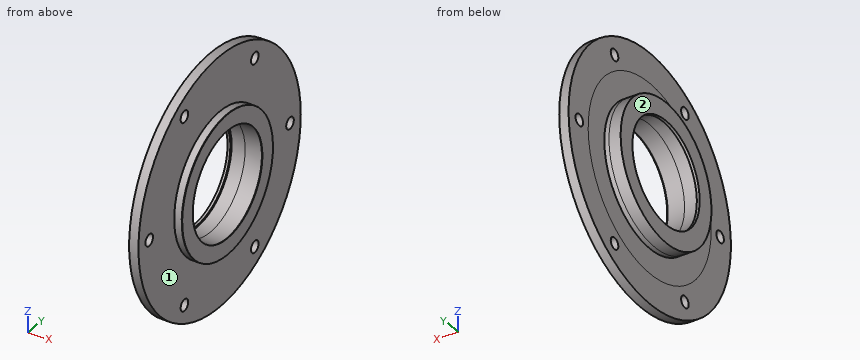
Autodesk Inventor part; units mm, degrees
ref_plane "Work Plane1" through (-10, 0, 0) normal (-1, 0, 0) x (0, 0, 1)
ref_plane "YZ Plane" through (0, 0, 0) normal (1, 0, 0) x (0, 1, 0)
ref_plane "XZ Plane" through (0, 0, 0) normal (0, 1, 0) x (-1, 0, 0)
sketch "Sketch1" plane through (0, 0, 0) normal (1, 0, 0) x (0, 1, 0)
  circle A0 centre (0, 0) radius 268
  circle A1 centre (0, 0) radius 203.25
  circle A2 centre (0, 0) radius 232.5
  circle A3 centre (232.5, 0) radius 12.5
  circle A4 centre (116.25, 201.3509) radius 12.5
  circle A5 centre (-116.25, 201.3509) radius 12.5
  circle A6 centre (-232.5, 0) radius 12.5
  circle A7 centre (-116.25, -201.3509) radius 12.5
  circle A8 centre (116.25, -201.3509) radius 12.5
  dimension "d2" = 465
  dimension "d0" = 536
  dimension "d1" = 406.5
  dimension "d3" = 25
  dimension "d101" = 360
extrude "Extrusion1" add sketch "Sketch1" along normal blind 20 contours A0 | A3 A2 A8 A7 A6 A5 A4
sketch "Sketch2" plane through (0, 0, 0) normal (1, 0, 0) x (0, 1, 0)
  circle A0 centre (0, 0) radius 115
  circle A1 centre (0, 0) radius 150
  dimension "d10" = 230
  dimension "d11" = 300
extrude "Extrusion2" add sketch "Sketch2" against normal mid plane 70
ref_plane "Work Plane1" through (-10, 0, 0) normal (-1, 0, 0) x (0, 0, 1)
sketch "Sketch3" plane through (-10, 0, 0) normal (-1, 0, 0) x (0, 0, 1)
  circle A0 centre (0, 0) radius 203.25
  circle A1 centre (0, 0) radius 150
  dimension "d15" = 406.5
  dimension "d16" = 300
extrude "Extrusion3" add sketch "Sketch3" against normal blind 30
sketch "Sketch4" plane through (-35, 0, 0) normal (-1, 0, 0) x (0, 0, 1)
  circle A0 centre (0, 0) radius 113.4667
  circle A1 centre (0, 0) radius 111
  circle A2 centre (0, 0) radius 115
  dimension "d43" = 222
  dimension "d44" = 230
extrude "Extrusion4" add sketch "Sketch4" against normal blind 6 contours A0 | A2
sketch "Sketch6" plane through (35, 0, 0) normal (1, 0, 0) x (0, 0, -1)
  circle A0 centre (0, 0) radius 150
  circle A1 centre (0, 0) radius 115
  dimension "d61" = 300
extrude "Extrusion6" add sketch "Sketch6" along normal blind 2.07
thread "Thread20"
sketch "Sketch9" plane through (-10, 0, 0) normal (-1, 0, 0) x (0, 0, 1)
  circle A0 centre (0, 0) radius 203.25
  circle A1 centre (0, 0) radius 150
extrude "Extrusion8" cut sketch "Sketch9" against normal up to surface (10 mm away)
thread "Thread30"
thread "Thread31"
thread "Thread32"
thread "Thread33"
thread "Thread34"
equation "\"BendRadius\" = Thickness"
equation "\"BendReliefWidth\" = Thickness"
equation "\"BendReliefDepth\" = 0.5 * Thickness"
equation "\"CornerReliefSize\" = 4 * Thickness"
equation "\"MinimumRemnant\" = 2 * Thickness"
equation "\"TransitionRadius\" = BendRadius"
equation "\"JacobiRadiusSize\" = BendRadius"
equation "\"GapSize\" = Thickness"
properties part number "elasmaROyleman"
Read the model definition and answer for the solid it produces. Units are mm, in the model's axes. Face numbers are marked on the shaded views. A direction names the side the tool comes from. Coordinates: 2 decimals unless noted, no trailing zeros. Order: outer loops, then holes, each group sorted by start corner. A loop starts at its lowest first (then second) coordinate and runs counter-clockwise, first axis right, second up. Notation, with made-up numbers: (28, -24) - (74, -24) arc R16 ccw to (74, 3) - close; hole circle Ø7 at (30, 41.25). An arc over 180 degrees is marked (long way). Answer as a JSON object with one key per item and string values. Group by question number.
Item 1: A tool of negligible diameter and unlimited length cuts with its end or side. For the marked faces 1 and 2, from which of +Z, -Z, +X, -X, +Y, -Y can it reach the whole face along a straight path? Write none if from no direction.
Item 2: Section C-C (z = 89.5) is taken. Give the vertices of the cut face in (x, y).
Item 3: Section B-B (z = 0) is taken. Give the vertices of the cut face in (x, y).
Item 4: Consider probe 1 along Y at (x, z) = (24, 0); probe 2 along Z at (x, y) = (7, 0); probe 3 along Z at (x, y) = (4, -3). Determine where each line is inside the solid, lowest interval first. Write a range as from..to.
Item 5: Section D-D (y = -138) is taken. Give the vertices of the cut face in (x, z).
Item 6: Flat-ended cylindrical pins translate along their axes: P1, Ø1.5, axis at x = -1.5, z = -151.5, coming from the +Y side; P2, Ø3, axis at x = -5.5, z = -30, coming from the -Y side; P3, Ø1, axis at x = -19.5, y = 19.5, coming from the +Z side; P4, Ø5, axis at x = 3.5, z = 161.5, coming from the -Y side. Find the tip coordinate at first contact, or state that the pin passes through.
Item 7: Section A-A (y = 0) is taken. Give the vertices of the cut face in (x, z).
Results are:
{
 "1": {"face 1": "+X", "face 2": "+Z, -Z, -X, +Y, -Y"},
 "2": {"outline": "(-35, -120.37) - (0, -120.37) - (0, -252.61) - (20, -252.61) - (20, -120.37) - (37.07, -120.37) - (37.07, -72.21) - (-29, -72.21) - (-29, -65.66) - (-35, -65.66) - close; (-35, 65.66) - (-29, 65.66) - (-29, 72.21) - (37.07, 72.21) - (37.07, 120.37) - (20, 120.37) - (20, 252.61) - (0, 252.61) - (0, 120.37) - (-35, 120.37) - close"},
 "3": {"outline": "(-35, -150) - (0, -150) - (0, -220) - (20, -220) - (20, -150) - (37.07, -150) - (37.07, -115) - (-29, -115) - (-29, -111) - (-35, -111) - close; (-35, 111) - (-29, 111) - (-29, 115) - (37.07, 115) - (37.07, 150) - (20, 150) - (20, 220) - (0, 220) - (0, 150) - (-35, 150) - close; (0, -268) - (20, -268) - (20, -245) - (0, -245) - close; (0, 245) - (20, 245) - (20, 268) - (0, 268) - close"},
 "4": {"probe 1": "y = -150..-115, 115..150", "probe 2": "z = -268..-115, 115..268", "probe 3": "z = -267.98..-114.96, 114.96..267.98"},
 "5": {"outline": "(-35, -58.79) - (0, -58.79) - (0, -229.74) - (20, -229.74) - (20, -58.79) - (37.07, -58.79) - (37.07, 58.79) - (20, 58.79) - (20, 229.74) - (0, 229.74) - (0, 58.79) - (-35, 58.79) - close"},
 "6": {"P1": "passes through", "P2": "stops at y = -147.27", "P3": "stops at z = 148.79", "P4": "stops at y = -215.74"},
 "7": {"outline": "(-35, -150) - (0, -150) - (0, -268) - (20, -268) - (20, -150) - (37.07, -150) - (37.07, -115) - (-29, -115) - (-29, -111) - (-35, -111) - close; (-35, 111) - (-29, 111) - (-29, 115) - (37.07, 115) - (37.07, 150) - (20, 150) - (20, 268) - (0, 268) - (0, 150) - (-35, 150) - close"}
}
